Build history of the part. All positions in model axes, mm. Round coordinates to 2 decimals unless told otherwise and drop trailing zeros. Order: outer loops, then holes, each group sorted by start corner. A loop starts at its lowest first (then second) coordinate and runs counter-clockwise, first axis right, second up. Notation, with made-up numbers: M 37.5,-22 L 64.5,-22 A19 cw 64.5,-3 Z; hole C 8,7 d11. An arc over 180 degrees is marked long. Use CSV: the item, a comma, the result in double quotes.
from build123d import *

# Parameters (mm, degrees)
BOSS_EXTRUDE1_DEPTH = 5
SKETCH2_R           = 6.35
CUT_EXTRUDE1_DEPTH  = 11
SKETCH3_OUTSIDE_W   = 73.518
SKETCH3_OUTSIDE_H   = 77.448
SKETCH3_OUTSIDE_R   = 12.7
CUT_EXTRUDE2_DEPTH  = 11
CUT_EXTRUDE2_TAPER  = 60


with BuildPart() as part:
    # Sketch1 → Boss-Extrude1 (new body, symmetric)
    with BuildSketch(Plane(origin=(0, 0, 0), x_dir=(1, 0, 0), z_dir=(0, 1, 0))):
        Polygon((-12.7, -7.332348419), (0, -14.664696837), (12.7, -7.332348419), (12.7, 7.332348419), (0, 14.664696837), (-12.7, 7.332348419), align=None)
    extrude(amount=BOSS_EXTRUDE1_DEPTH, both=True)

    # Sketch2 → Cut-Extrude1 (cut, through all)
    with BuildSketch(Plane(origin=(0, 5, 0), x_dir=(1, 0, 0), z_dir=(0, 1, 0))):
        Circle(SKETCH2_R)
    extrude(amount=-CUT_EXTRUDE1_DEPTH, mode=Mode.SUBTRACT)

    # Sketch3 outside → Cut-Extrude2 (cut, through all)
    with BuildSketch(Plane(origin=(0, 5, 0), x_dir=(1, 0, 0), z_dir=(0, 1, 0))):
        Rectangle(SKETCH3_OUTSIDE_W, SKETCH3_OUTSIDE_H)
        Circle(SKETCH3_OUTSIDE_R, mode=Mode.SUBTRACT)
    cut_extrude2 = extrude(amount=-CUT_EXTRUDE2_DEPTH, taper=CUT_EXTRUDE2_TAPER, mode=Mode.SUBTRACT)

    # Mirror1: Cut-Extrude2 across plane
    add(cut_extrude2.mirror(Plane.ZX), mode=Mode.SUBTRACT)


solid = part.part
(1) Drop a flat-ended pin along its axis: pin 1 (5 mm diameter, centred on x = -4.5, y = -2.5, fed in from +Z). Give the stop position or say it passes through.
Answer block:
pin 1,"stops at z = 13.51"
(2) Cut at B-B, the plane y = -4.5. Give the cut face in (x, z), and give its area (3 significant figures).
Answer block:
outline,"M -12.7,-4.77 A13.57 ccw -10.48,-8.61 L -2.22,-13.38 A13.57 ccw 2.22,-13.38 L 10.48,-8.61 A13.57 ccw 12.7,-4.77 L 12.7,4.77 A13.57 ccw 10.48,8.61 L 2.22,13.38 A13.57 ccw -2.22,13.38 L -10.48,8.61 A13.57 ccw -12.7,4.77 Z; hole C 0,0 d12.7"
area,"418 mm²"
(3) Cut at A-A, the plane y = 3.5. Give the cut face in (x, z), and give its area (3 significant figures).
Answer block:
outline,"M -12.7,-7.33 L 0,-14.66 L 12.7,-7.33 L 12.7,7.33 L 0,14.66 L -12.7,7.33 Z; hole C 0,0 d12.7"
area,"432 mm²"
(4) Two-plate mould, pull along Z, no slides. Class faces 1 (the face through (-1.38, 0.07, 6.2)), 2 (the face through (0.032, 4.724, 13.178)), 3 (the face through (11.4, 4.72, -6.62)), 4 (the face through (-12.7, 0, 0)): released by +Z, released by -Z, zero draft, split by the parting line, or undercut.
Answer block:
face 1,"undercut"
face 2,"released by +Z"
face 3,"released by -Z"
face 4,"zero draft"
(5) Wall check: line 1 (X direction, y = 2.25, z = 0); line 2 (Z direction, x = 2, y = 3.25); line 3 (Z direction, x = 3, y = 4). Give the ranges that are in metal, low to high. Write a range as from..to.
Answer block:
line 1,"x = -12.7..-6.35, 6.35..12.7"
line 2,"z = -13.51..-6.03, 6.03..13.51"
line 3,"z = -12.93..-5.6, 5.6..12.93"
